from build123d import *

# Parameters (mm, degrees)
EXTRUDE_1_DEPTH = 14


with BuildPart() as part:
    # Эскиз1 → Бобышка-Вытянуть1 (new body)
    with BuildSketch(Plane(origin=(0, 0, 0), x_dir=(1, 0, 0), z_dir=(0, 1, 0))):
        Polygon((-8.660254038, 15), (-17.320508076, 0), (-8.660254038, -15), (8.660254038, -15), (17.320508076, 0), (8.660254038, 15), align=None)
    extrude(amount=EXTRUDE_1_DEPTH)

    # Эскиз2 → Вырез-Повернуть1 (revolve, cut)
    with BuildSketch(Plane(origin=(0, 0, 0), x_dir=(0, 0, -1), z_dir=(1, 0, 0))):
        Polygon((-15, 14), (-20, 14), (-20, 11.113248654), align=None)
        Polygon((-15, 0), (-20, 0), (-20, 2.886751346), align=None)
    revolve(axis=Axis((0, -1000, 0), (0, 1, 0)), mode=Mode.SUBTRACT)

    # Эскиз3 → Отверстие обработанное метчиком M20x2.51 (revolve, cut)
    with BuildSketch(Plane(origin=(0, 0, 0), x_dir=(0, 0, -1), z_dir=(1, 0, 0))):
        Polygon((0, 0), (0, 14), (10.025, 14), (8.75, 12.725), (8.75, 1.275), (10.025, 0), align=None)
    revolve(axis=Axis((0, -6.35, 0), (0, 1, 0)), mode=Mode.SUBTRACT)


solid = part.part
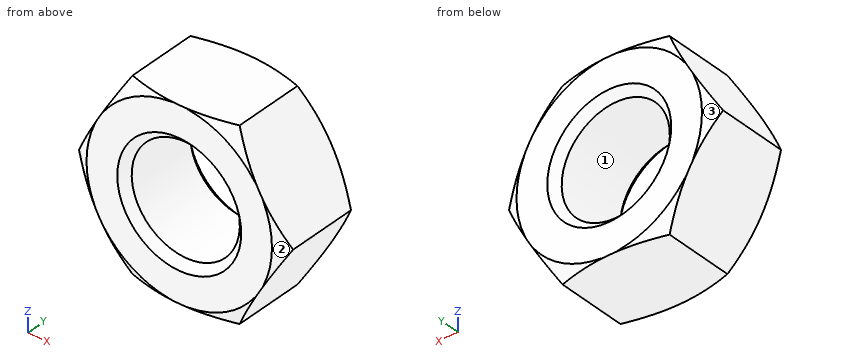
Could you check a few things on this model? Use its own coordinates, in mm. Face numbers are marked on the shaded views. Give positions to 0.01 mm unless a question says otherwise; leave off trailing zeros. Loops run counter-clockwise (first coordinate to the right, second up) from the corner with the lowest first, then second, coordinate; pieces in that order, holes last. Notation, with made-up numbers: M 29.25,6 L 41.25,6 A28 cw 41.25,35 Z; hole C 77,-23 d11. An arc over 180 degrees is marked long. Answer as a JSON object with one key per item and string values.
Q1. If I drill on probe 1 along X at (y, z) = (7.5, 0); probe 2 along Z at (x, y) = (4.5, 4.5); probe 3 along Z at (x, y) = (0.5, 8), over which ranges is the centre line in solid material (lowest first)? Write a range as [from, to].
Values found:
{"probe 1": "x = [-17.32, -8.75], [8.75, 17.32]", "probe 2": "z = [-15, -7.5], [7.5, 15]", "probe 3": "z = [-15, -8.74], [8.74, 15]"}
Q2. For P1, Ø1, axis at y = 8.5, z = -4, coming from the +X side; P2, Ø1, axis at y = 4, z = -8.5, coming from the +X side; P3, Ø8, axis at x = -14, y = 5.5, coming from the +Z side; P4, Ø3, axis at x = 4, z = 11.5, coming from the -Y side, each with a flat end and sliding along its axis, tell me the tip position at first contact or that it passes through.
Values found:
{"P1": "stops at x = 15.3", "P2": "stops at x = 12.7", "P3": "stops at z = 12.68", "P4": "stops at y = 0"}
Q3. Suppose I cut it at A-A, the plane y = 5.25. List the corners of the cut face in (x, z) for me, plus the area to 3 significant figures.
Values found:
{"outline": "M -17.32,0 L -8.66,-15 L 8.66,-15 L 17.32,0 L 8.66,15 L -8.66,15 Z; hole C 0,0 d17.5", "area": "539 mm²"}
Q4. Suppose I cut it at B-B, the plane y = 13.25. List the corners of the cut face in (x, z) for me (3 decimals), plus the area to 3 significant figures.
Values found:
{"outline": "M -16.179,-1.978 L -9.802,-13.022 A16.299 ccw -6.376,-15 L 6.376,-15 A16.299 ccw 9.802,-13.022 L 16.179,-1.978 A16.299 ccw 16.179,1.978 L 9.802,13.022 A16.299 ccw 6.376,15 L -6.376,15 A16.299 ccw -9.802,13.022 L -16.179,1.978 A16.299 ccw Z; hole C 0,0 d18.55", "area": "498 mm²"}
Q5. If we mould it in two halves opening along X, with no side actions, what happens to the marked faces 1, 2 and 3? For each: pulls with the +X half, pulls with the -X half, needs draft (parallel to the pull), parting line crosses it, or undercut.
Values found:
{"face 1": "undercut", "face 2": "pulls with the +X half", "face 3": "pulls with the -X half"}
